Geometry check sheet. Reference: drawing and pictorial views, mm from the part's lowest x, y, z. A direction names the side the tool comes from. Round coordinates to 2 decimals unless told otherwise and drop trailing zeros. Order: outer loops, then holes, each group sorted by start corner. A loop starts at its lowest first (then second) coordinate and runs counter-clockwise, first axis right, second up.
(1) Sectioned sample at D-D (y = 17). Record the boundary of the cut face in (x, z) (1 decimal).
(2) Sectioned sample at A-A (z = 0.8). Record the boundary of the cut face in (x, y) (1 decimal), plus the area to 3 significant figures.
(3) Sectioned sample at B-B (x = 12.5). Record the boundary of the cut face in (y, z) (1 decimal).
(4) Release check for a two-part mould opening along X. For the marked faces 1, 2 and 3 record: +X half, -X half, draft (parallel to the pull), parting line (faces both ways), or undercut.
(5) Set-up check for the marked faces 4 and 5: record each of +Z, -Z, +X, -X, +Y, -Y from which the full face is reachable in a straight line by a thin tool's end or side.
(6) Material ranges on line 1 along X through (y, z) = (11.25, 1.3) (1 decimal); line 2 along Y through (x, z) = (14.5, 0.25) (1 decimal); line 3 along X through (y, z) = (10.25, 0.2) (1 decimal), recorded low to high.
(7) Go/stop test with a flat-tipped pin: pin 1 (2 mm diameter, centred on x = 6.5, y = 8, fed in from +Z). Record where the tip stops, or that it passes through.
(8) Sectioned sample at C-C (y = 7.25). Record the boundary of the cut face in (x, z).
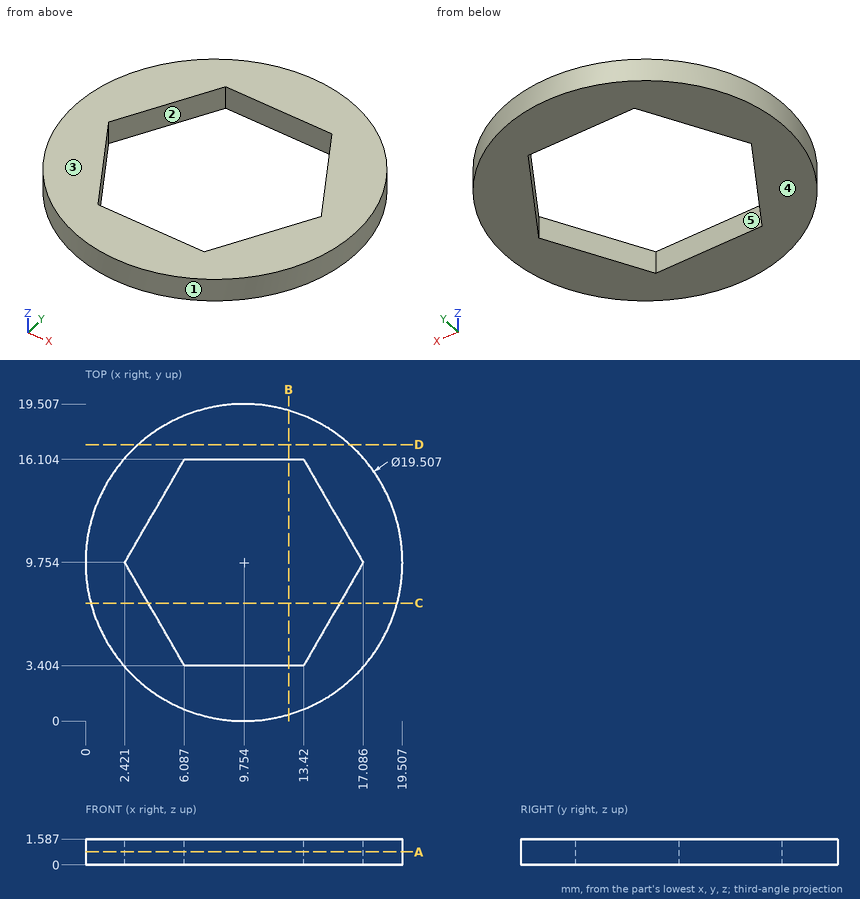
Answer below:
1. outline: (3.2, 0) - (16.3, 0) - (16.3, 1.6) - (3.2, 1.6) - close
2. outline: circle Ø19.5 at (9.8, 9.8); hole (2.4, 9.8) - (6.1, 3.4) - (13.4, 3.4) - (17.1, 9.8) - (13.4, 16.1) - (6.1, 16.1) - close
2. area: 159 mm2
3. outline: (0.4, 0) - (3.4, 0) - (3.4, 1.6) - (0.4, 1.6) - close; (16.1, 0) - (19.1, 0) - (19.1, 1.6) - (16.1, 1.6) - close
4. face 1: parting line
4. face 2: undercut
4. face 3: draft
5. face 4: -Z, +X, -X, +Y, -Y
5. face 5: +Z, -Z
6. line 1: x = 0.1 to 3.3, 16.2 to 19.4
6. line 2: y = 1.2 to 5.3, 14.2 to 18.3
6. line 3: x = 0 to 2.7, 16.8 to 19.5
7. pin 1: passes through
8. outline: (0.33, 0) - (3.87, 0) - (3.87, 1.59) - (0.33, 1.59) - close; (15.64, 0) - (19.18, 0) - (19.18, 1.59) - (15.64, 1.59) - close
